Answer from the drawing. Dimensions are ordinates in mm from the lowest x, y and z of the part. A direction names the side the tool comes from. Coordinates: 2 decimals unless noted, no trailing zeros. Write each loop counter-clockwise with the first axis right and the second up, starting at its lowest first coordinate (ties: lowest second). Pieces come first, ordered by that corner, then holes. Notation, with made-up numbers: (12.5, -13.75) - (65.5, -13.75) arc R23 ccw to (65.5, 3.25) - close; hole circle Ø9 at (87.25, -16.5). An arc over 180 degrees is marked (long way). Use a Markdown table: item, result.
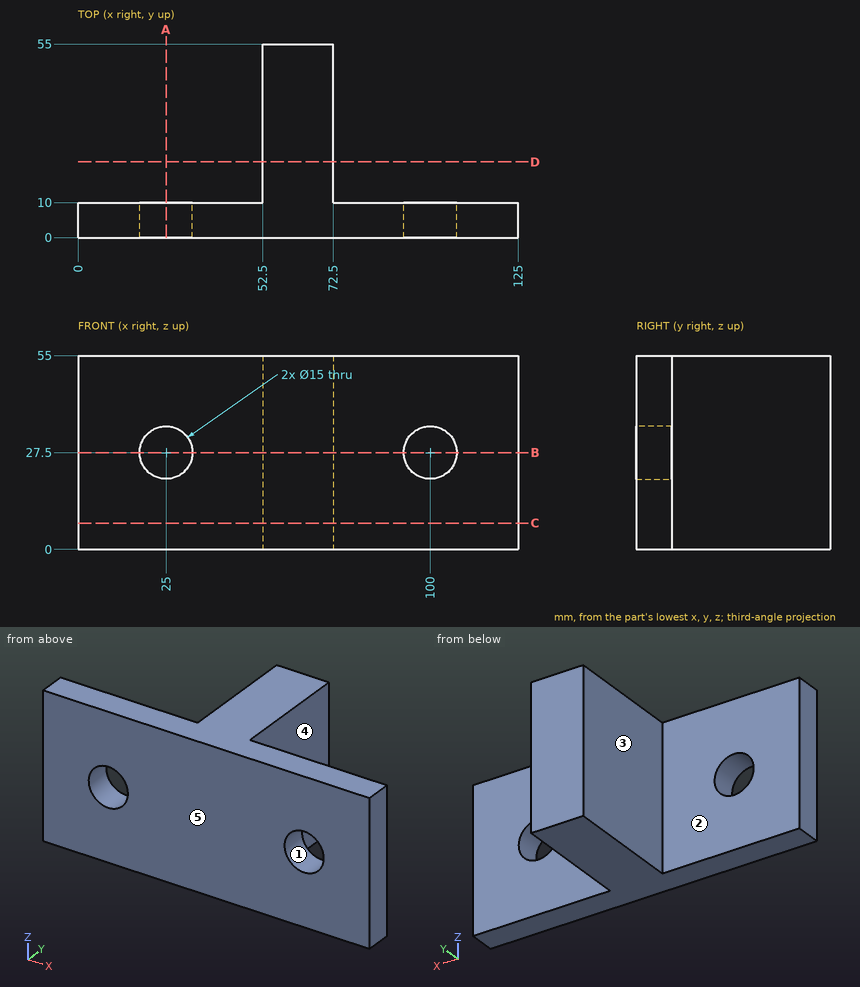
(1) Straight lines are drawn through the part: L1, parallel to X at y = 2.5, z = 27.5; L2, parallel to Y at x = 116, z = 43.5; L3, parallel to X at y = 31.5, z = 40.5. For each, find the intervals that lie inside material, in ascending order.
Report:
| item | result |
|---|---|
| L1 | x = 0 to 17.5, 32.5 to 92.5, 107.5 to 125 |
| L2 | y = 0 to 10 |
| L3 | x = 52.5 to 72.5 |
(2) Each of these flat-tipped pins is pushed along its axis until it touches: P1, Ø16, axis at x = 36.5, z = 31, coming from the +Y side; P2, Ø10, axis at y = 22.5, z = 39.5, coming from the +X side. Where does it stop, or does it pass through?
Report:
| item | result |
|---|---|
| P1 | stops at y = 10 |
| P2 | stops at x = 72.5 |
(3) The mould has two halves that part along X. Classify the marked faces 1, 2 and 3: pulls with the +X half, pulls with the -X half, needs draft (parallel to the pull), parting line crosses it, or undercut.
Report:
| item | result |
|---|---|
| face 1 | undercut |
| face 2 | needs draft |
| face 3 | pulls with the -X half |
(4) A cutting plane is placed at A-A, the plane x = 25. Write down the section's boundary in (y, z).
Report:
| item | result |
|---|---|
| outline | (0, 0) - (10, 0) - (10, 20) - (0, 20) - close; (0, 35) - (10, 35) - (10, 55) - (0, 55) - close |
(5) For the marked faces 4 and 5, determine the directions among +Z, -Z, +X, -X, +Y, -Y from which every point of the face is accessible in a straight line to the end or side of a thin tool.
Report:
| item | result |
|---|---|
| face 4 | +Z, -Z, +X, +Y |
| face 5 | +Z, -Z, +X, -X, -Y |
(6) A cutting plane is placed at D-D, the plane y = 21.5. Write down the section's boundary in (x, z).
Report:
| item | result |
|---|---|
| outline | (52.5, 0) - (72.5, 0) - (72.5, 55) - (52.5, 55) - close |
(7) A cutting plane is placed at B-B, the plane z = 27.5. Write down the section's boundary in (x, y).
Report:
| item | result |
|---|---|
| outline | (0, 0) - (17.5, 0) - (17.5, 10) - (0, 10) - close; (32.5, 0) - (92.5, 0) - (92.5, 10) - (72.5, 10) - (72.5, 55) - (52.5, 55) - (52.5, 10) - (32.5, 10) - close; (107.5, 0) - (125, 0) - (125, 10) - (107.5, 10) - close |
(8) A cutting plane is placed at C-C, the plane z = 7.5. Write down the section's boundary in (x, y).
Report:
| item | result |
|---|---|
| outline | (0, 0) - (125, 0) - (125, 10) - (72.5, 10) - (72.5, 55) - (52.5, 55) - (52.5, 10) - (0, 10) - close |
